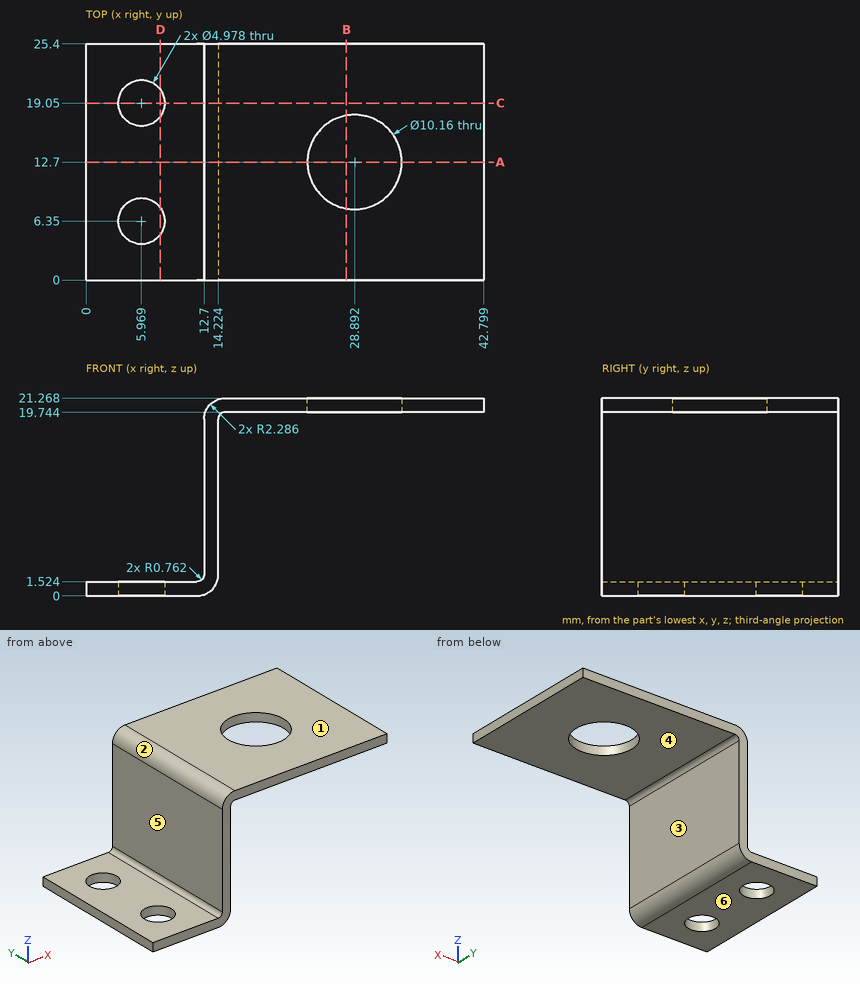
Could you check a few things on this drawing? It's one solid part, dimensions in mm from its lowest x, y, z. A direction names the side the tool comes from. Give positions to 0.01 mm unless a question says otherwise; leave off trailing zeros. Loops run counter-clockwise (first coordinate to the right, second up) from the corner with the lowest first, then second, coordinate; pieces in that order, holes last. Notation, with made-up numbers: (-21.5, 0.5) -> (25.5, 0.5) arc R20 ccw to (25.5, 32.5) -> close; hole circle Ø4 at (4.5, 43). An arc over 180 degrees is marked (long way). Use one line per item in the form item = value. Start each with the question number.
1) Thinking about a two-plate mould opening in X: for the marked faces 1, 2 and 3, which applies, +X half, -X half, draft (parallel to the pull), parting line (faces both ways), or undercut?
2) Which directions (+Z, -Z, +X, -X, +Y, -Y) give clear straight access to the entire face, cutting with the end or side of a thin tool? Please do the marked faces 4, 5 and 6.
3) Imagine slicing it at C-C (y = 19.05). Please give me the cut outline in (x, z) (1 decimal).
4) For P1, Ø7.5, axis at x = 27, y = 14.5, coming from the -Z side; P2, Ø4, axis at x = 14.5, y = 6.5, coming from the -Z side; P3, Ø2, axis at y = 20, z = 19, coming from the -X side; P4, Ø8, axis at x = 28.89, y = 12.7, coming from the -Z side, each with a flat end and sliding along its axis, tell me the tip position at first contact or that it passes through.
5) Please list where these lines run through material, in increasing order: line 1 along Z through (x, y) = (16.5, 6.25) (1 decimal); line 2 along X through (y, z) = (12.25, 18.25) (1 decimal); line 3 along Z through (x, y) = (10.5, 6.25) (1 decimal).
6) Imagine slicing it at D-D (x = 8). Please give me the cut outline in (y, z) (1 decimal).
7) Imagine slicing it at A-A (y = 12.7). Please give me the cut outline in (x, z) (1 decimal).
8) Imagine slicing it at B-B (x = 28). Please give me the cut outline in (y, z) (1 decimal).
Check values:
q1.face_1 = draft
q1.face_2 = -X half
q1.face_3 = +X half
q2.face_4 = -Z, +X, +Y, -Y
q2.face_5 = +Z, -X, +Y, -Y
q2.face_6 = -Z, +X, -X, +Y, -Y
q3.outline = (0, 0) -> (3.5, 0) -> (3.5, 1.5) -> (0, 1.5) -> close; (8.5, 0) -> (11.9, 0) arc R2.3 ccw to (14.2, 2.3) -> (14.2, 19) arc R0.8 cw to (15, 19.7) -> (42.8, 19.7) -> (42.8, 21.3) -> (15, 21.3) arc R2.3 ccw to (12.7, 19) -> (12.7, 2.3) arc R0.8 cw to (11.9, 1.5) -> (8.5, 1.5) -> close
q4.P1 = 19.74
q4.P2 = 0.07
q4.P3 = 12.7
q4.P4 = through
q5.line_1 = 19.7 to 21.3
q5.line_2 = 12.7 to 14.2
q5.line_3 = 0 to 1.5
q6.outline = (0, 0) -> (4.9, 0) -> (4.9, 1.5) -> (0, 1.5) -> close; (7.8, 0) -> (17.6, 0) -> (17.6, 1.5) -> (7.8, 1.5) -> close; (20.5, 0) -> (25.4, 0) -> (25.4, 1.5) -> (20.5, 1.5) -> close
q7.outline = (0, 0) -> (11.9, 0) arc R2.3 ccw to (14.2, 2.3) -> (14.2, 19) arc R0.8 cw to (15, 19.7) -> (23.8, 19.7) -> (23.8, 21.3) -> (15, 21.3) arc R2.3 ccw to (12.7, 19) -> (12.7, 2.3) arc R0.8 cw to (11.9, 1.5) -> (0, 1.5) -> close; (34, 19.7) -> (42.8, 19.7) -> (42.8, 21.3) -> (34, 21.3) -> close
q8.outline = (0, 19.7) -> (7.7, 19.7) -> (7.7, 21.3) -> (0, 21.3) -> close; (17.7, 19.7) -> (25.4, 19.7) -> (25.4, 21.3) -> (17.7, 21.3) -> close
